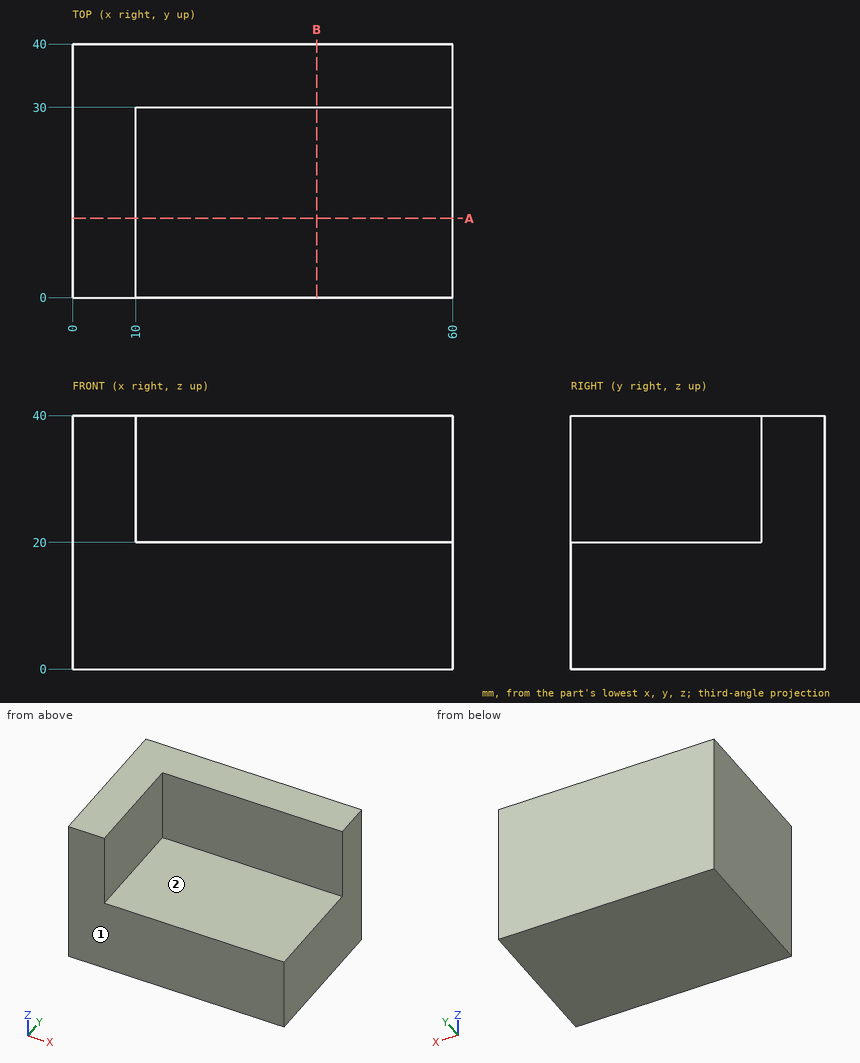
The figure shows three views and two pictorial views of one solid part (mm, origin at its lowest corner). Answer the questions. A direction names the side the tool comes from. Coordinates: 2 decimals unless noted, no trailing zeros. Write each loop counter-clockwise with the first axis right and the second up, starting at its lowest first coordinate (ties: lowest second). Pieces come first, ordered by that corner, then holes. Notation, with made-up numbers: (-6.5, 77) -> (6.5, 77) arc R16 cw to (6.5, 99) -> close; hole circle Ø11 at (-19, -1). An arc over 180 degrees is marked (long way). Answer as a JSON object with one key per item and string values.
Q1. Consider line 1 (Z direction, x = 20, y = 21); line 2 (X direction, y = 4, z = 21); line 3 (Y direction, x = 17, z = 21). Determine where each line is inside the solid, lowest interval first. Write a range as [from, to].
The answers:
{"line 1": "z = [0, 20]", "line 2": "x = [0, 10]", "line 3": "y = [30, 40]"}
Q2. The part is cut by section A-A on y = 12.5. Give the vertices of the cut face in (x, z).
The answers:
{"outline": "(0, 0) -> (60, 0) -> (60, 20) -> (10, 20) -> (10, 40) -> (0, 40) -> close"}
Q3. A tool of negligible diameter and unlimited length cuts with its end or side. For the marked faces 1 and 2, from which of +Z, -Z, +X, -X, +Y, -Y can it reach the whole face along a straight path? Write none if from no direction.
The answers:
{"face 1": "+Z, -Z, +X, -X, -Y", "face 2": "+Z, +X, -Y"}
Q4. Flat-ended cylindrical pins translate along their axes: pin 1 Ø10 at (x, y) = (54, 9.5) entering from +Z; pin 2 Ø16 at (x, z) = (46.5, 28.5) entering from -Y. Find the tip coordinate at first contact, or state that the pin passes through.
The answers:
{"pin 1": "stops at z = 20", "pin 2": "stops at y = 30"}
Q5. The part is cut by section B-B on x = 38.5. Give the vertices of the cut face in (y, z).
The answers:
{"outline": "(0, 0) -> (40, 0) -> (40, 40) -> (30, 40) -> (30, 20) -> (0, 20) -> close"}
